Geometry check sheet. Reference: the model listing, model coordinates, mm. A direction names the side the tool comes from. Coordinates: 2 decimals unless noted, no trailing zeros. Write each loop counter-clockwise with the first axis right and the second up, starting at its lowest first coordinate (ties: lowest second). Pieces come first, ordered by that corner, then holes. Notation, with made-up numbers: (-14, 11) -> (10, 11) arc R19 cw to (10, 34) -> close; hole circle Ø2 at (-34, 28.5). An arc over 180 degrees is marked (long way). Use a Markdown table: item, result.
```python
from build123d import *

# Parameters (mm, degrees)
F0_W     = 1.6891
F0_H     = 1.56845
F0_H_2   = 1.6891
F0_W_2   = 1.56845
F1_DEPTH = 39.6875
F2_R     = 2.54
F3_DEPTH = 35.71875


with BuildPart() as f1:
    # F0 (on Top) → F1 (new body, symmetric)
    with BuildSketch(Plane.XY):
        with Locations((0, -1.628775)):
            Rectangle(F0_W, F0_H)
        Rectangle(F0_W, F0_H_2)
        with Locations((1.628775, 0)):
            Rectangle(F0_W_2, F0_H_2)
        with Locations((-1.628775, 0)):
            Rectangle(F0_W_2, F0_H_2)
        with Locations((0, 1.628775)):
            Rectangle(F0_W, F0_H)
    extrude(amount=F1_DEPTH, both=True)

    # F2 (on Top) → F3 (join, symmetric)
    with BuildSketch(Plane.XY):
        Circle(F2_R)
    extrude(amount=F3_DEPTH, both=True)


solid = f1.part
```
Item 1: Thickness scan on L1, parallel to Z at x = 1.4, y = 1.45; L2, parallel to X at y = -0.75, z = 27.5; L3, parallel to X at y = 2.3, z = -11.5. Record the ranges inside material, lowest first. Write a range as [from, to].
Answer block:
| item | result |
|---|---|
| L1 | z = [-35.72, 35.72] |
| L2 | x = [-2.43, 2.43] |
| L3 | x = [-1.08, 1.08] |
Item 2: Tool access check on faces 1 (the flat face through (-0.845, 2, 38)), 2 (the flat face through (-1, -1, 35.719)), 3 (the flat face through (-1, 1, -35.719)), 4 (the flat face through (-0.845, -2, 38)), 5 (the flat face through (2, 0.845, 38)). Record the directions out of +Z, -Z, +X, -X, +Y, -Y that give a thin tool (end or side, any length) a straight path to the whole face; none if there is none.
Answer block:
| item | result |
|---|---|
| face 1 | -X, +Y |
| face 2 | +Z, -X, -Y |
| face 3 | -Z, -X, +Y |
| face 4 | -X, -Y |
| face 5 | +X, +Y |
Item 3: Section check B-B on y = 1.5. Record the boundary of the cut face in (x, z), then the cut area to 3 significant figures.
Answer block:
| item | result |
|---|---|
| outline | (-2.05, -35.72) -> (-0.84, -35.72) -> (-0.84, -39.69) -> (0.84, -39.69) -> (0.84, -35.72) -> (2.05, -35.72) -> (2.05, 35.72) -> (0.84, 35.72) -> (0.84, 39.69) -> (-0.84, 39.69) -> (-0.84, 35.72) -> (-2.05, 35.72) -> close |
| area | 306 mm^2 |
Item 4: Depth check by flat-ended pin: P1, Ø0.8, axis at y = 1.5, z = 13, coming from the -X side; P2, Ø1, axis at x = -1.5, z = 7.5, coming from the -Y side; P3, Ø0.5, axis at x = -1.5, y = 1.5, coming from the +Z side. Enter the tip coordinate at first touch or a pass-through.
Answer block:
| item | result |
|---|---|
| P1 | stops at x = -2.29 |
| P2 | stops at y = -2.33 |
| P3 | stops at z = 35.72 |
Item 5: Section check C-C on y = -1.55. Record the boundary of the cut face in (x, z).
Answer block:
| item | result |
|---|---|
| outline | (-2.01, -35.72) -> (-0.84, -35.72) -> (-0.84, -39.69) -> (0.84, -39.69) -> (0.84, -35.72) -> (2.01, -35.72) -> (2.01, 35.72) -> (0.84, 35.72) -> (0.84, 39.69) -> (-0.84, 39.69) -> (-0.84, 35.72) -> (-2.01, 35.72) -> close |
